Verification items for the finished model (mm, model axes). A direction names the side the tool comes from. Give positions to 0.01 mm unless a question says otherwise; leave off trailing zeros. Write each loop counter-clockwise with the first axis right and the second up, starting at its lowest first coordinate (ties: lowest second). Pieces come first, ordered by that corner, then holes. Notation, with made-up numbers: (-5.75, 0.25) -> (42.25, 0.25) arc R26 ccw to (42.25, 26.25) -> close; hole circle Ø5 at (30.5, -24). An arc over 180 degrees is marked (long way). Use one line per item in the form item = value. Start each with the question number.
(1) Section check B-B, the plane y = -2.75. Record the cut outline in (x, z), plus the area to 3 significant figures.
(2) Set-up check for faces 5 (the face through (26.471, -13, 3)), 6 (the face through (6.293, -12.878, 15.609)): record each of +Z, -Z, +X, -X, +Y, -Y from which the full face is reachable in a straight line by a thin tool's end or side.
(3) Depth check by flat-ended pin: pin 1 Ø10 at (x, y) = (21, -7.5) entering from -Z; pin 2 Ø5 at (y, z) = (-8.5, 3.5) entering from +X; pin 3 Ø6 at (x, y) = (4, -21) entering from +Z. Enter the tip coordinate at first touch or a pass-through.
(4) Scan lines: L1, parallel to X at y = -18.75, z = 2; L2, parallel to X at y = -3, z = 3; L3, parallel to Z at x = 24.5, y = -18.75. Record each from-to range of solid material in increasing order.
(5) Section check A-A, the plane z = 4. Record the cut outline in (x, y), plus the area to 3 significant figures.
(6) Release check for a two-part mould opening along X. For faces 1 (the face through (20, -13, 6.35)), 2 (the face through (13.771, -13, 3)), 3 (the face through (32, -13, 0)), 4 (the face through (31.773, -12.878, 16.053)) record: pulls with the +X half, pulls with the -X half, needs draft (parallel to the pull), parting line crosses it, or undercut.
(7) Section check D-D, the plane z = 20.5. Record the cut outline in (x, y).
(8) Section check C-C, the plane x = 34. Record the cut outline in (y, z).
from build123d import *

# Parameters (mm, degrees)
F0_W     = 38.2962413132
F0_H     = 31.662248075
F1_DEPTH = 25.4
F3_DEPTH = 25.401
F5_DEPTH = 25.4
F6_DEPTH = 50.801
F7_W     = 12.7
F7_H     = 6.35
F8_DEPTH = 25.4


with BuildPart() as f1:
    # F0 (on Front) → F1 (new body)
    with BuildSketch(Plane.XZ):
        with Locations((19.1481206566, 15.8311240375)):
            Rectangle(F0_W, F0_H)
    extrude(amount=F1_DEPTH)

    # F2 (on face) → F3 (cut, through all)
    with BuildSketch(Plane.XZ.offset(25.4)):
        Polygon((0, 31.662248075), (0, 0), (12.7654150128, 31.662248075), align=None)
    extrude(amount=-F3_DEPTH, mode=Mode.SUBTRACT)

    # F4 (on face) → F5 (join)
    with BuildSketch(Plane.XZ.offset(25.4)):
        Polygon((25.4303161055, 31.662248075), (38.2962413132, 0), (38.2962413132, 31.662248075), align=None)
    extrude(amount=F5_DEPTH)

    # F6 (cut, through all): a face of the model
    f6_faces = [f1.faces().sort_by_distance(p)[0] for p in [
        (34.0075995773, -50.8, 21.1081653833),
    ]]
    extrude(f6_faces, amount=-F6_DEPTH, mode=Mode.SUBTRACT)

    # F7 (on face) → F8 (cut)
    with BuildSketch(Plane.XZ.offset(25.4)):
        with Locations((20.1205644593, 3.175)):
            Rectangle(F7_W, F7_H)
    extrude(amount=-F8_DEPTH, mode=Mode.SUBTRACT)


solid = f1.part
Completed:
q1.outline = (0, 0) -> (13.77, 0) -> (13.77, 6.35) -> (26.47, 6.35) -> (26.47, 0) -> (38.3, 0) -> (25.43, 31.66) -> (12.77, 31.66) -> close
q1.area = 726 mm²
q2.face_5 = -Z, +Y, -Y
q2.face_6 = +Z, -X, +Y, -Y
q3.pin_1 = 6.35
q3.pin_2 = 37.89
q3.pin_3 = 17.36
q4.L1 = 0.81 to 13.77, 26.47 to 37.48
q4.L2 = 1.21 to 13.77, 26.47 to 37.08
q4.L3 = 6.35 to 31.66
q5.outline = (1.61, -25.4) -> (13.77, -25.4) -> (13.77, 0) -> (1.61, 0) -> close; (26.47, -25.4) -> (36.67, -25.4) -> (36.67, 0) -> (26.47, 0) -> close
q5.area = 568 mm²
q6.face_1 = undercut
q6.face_2 = undercut
q6.face_3 = needs draft
q6.face_4 = pulls with the +X half
q7.outline = (8.27, -25.4) -> (29.97, -25.4) -> (29.97, 0) -> (8.27, 0) -> close
q8.outline = (-25.4, 0) -> (0, 0) -> (0, 10.57) -> (-25.4, 10.57) -> close
